Verification items for the finished model (mm, model axes). Coordinates: 2 decimals unless noted, no trailing zeros. Loops run counter-clockwise (first coordinate to the right, second up) from the corner with the lowest first, then second, coordinate; pieces in that order, holes last. Notation, with made-up numbers: (34.25, 61) - (73.25, 61) arc R18 ccw to (73.25, 81) - close; hole circle Ø6 at (61.25, 77). An arc over 180 degrees is marked (long way). One line per item, written item: value. Start each with the question number.
(1) Section check C-C (y = 0). Record the boundary of the cut face in (x, z).
(2) Draft check along X on faces 1 (the face through (-1, -35, 1)), 2 (the face through (-34.136, -1.187, 1.521)), 3 (the face through (-22.387, 18, 2)). Enter one of: +X half, -X half, draft (parallel to the pull), parting line (faces both ways), or undercut.
(3) Thickness scan on probe 1 along X at (y, z) = (-16.5, 0.85); probe 2 along Y at (x, z) = (-37, 1.05); probe 3 along Y at (x, z) = (0, 1.9). Record the ranges inside material, lowest first. Write a range as [from, to].
(4) Section check D-D (x = -32.5). Record the boundary of the cut face in (y, z), plus the area to 3 significant figures.
(5) Section check B-B (x = 13). Record the boundary of the cut face in (y, z), plus the area to 3 significant figures.
(6) Section check A-A (x = 31.5). Record the boundary of the cut face in (y, z).
(7) Gauge pin test, flat ends, axial feed: P1, Ø8, axis at x = -0.5, y = 8.5, coming from the -Z side; P2, Ø3.5, axis at x = -37, y = 0, coming from the +Z side. Record the tip position at first contact, or that the pin passes through.
```python
from build123d import *

# Parameters (mm, degrees)
SKETCH1_W               = 100
SKETCH1_H               = 70
BOSS_EXTRUDE1_DEPTH     = 3
SKETCH2_R               = 3.1
CUT_EXTRUDE1_DEPTH      = 62.10646447
SKETCH3_R               = 1.5
CUT_EXTRUDE2_DEPTH      = 62.10646447
MIRROR2_COPY_1_SKETCH_R = 1.5
MIRROR2_COPY_1_DEPTH    = 62.10646447
CUT_EXTRUDE3_DEPTH      = 62.10646447


with BuildPart() as part:
    # Sketch1 → Boss-Extrude1 (new body)
    with BuildSketch(Plane.XY):
        Rectangle(SKETCH1_W, SKETCH1_H)
    extrude(amount=BOSS_EXTRUDE1_DEPTH)

    # Sketch2 → Cut-Extrude1 (cut, through all)
    with BuildSketch(Plane.XY.offset(3)):
        with Locations((-17, 0)):
            Circle(SKETCH2_R)
        with Locations((-37, 0)):
            Circle(SKETCH2_R)
        with Locations((13, 0)):
            Circle(SKETCH2_R)
    extrude(amount=-CUT_EXTRUDE1_DEPTH, mode=Mode.SUBTRACT)

    # Sketch3 → Cut-Extrude2 (cut, through all)
    with BuildSketch(Plane.XY.offset(3)):
        with Locations((-45.644550594, 30.644550594)):
            Circle(SKETCH3_R)
    cut_extrude2 = extrude(amount=-CUT_EXTRUDE2_DEPTH, mode=Mode.SUBTRACT)

    # Mirror1: Cut-Extrude2 across plane
    add(cut_extrude2.mirror(Plane(origin=(0, 0, 0), x_dir=(0, 0, 1), z_dir=(1, 0, 0))), mode=Mode.SUBTRACT)

    # Mirror2: Cut-Extrude2 across plane
    add(cut_extrude2.mirror(Plane.ZX), mode=Mode.SUBTRACT)

    # Mirror2 copy 1 sketch → Mirror2 copy 1 (cut, through all)
    with BuildSketch(Plane(origin=(0, 0, 3), x_dir=(-1, 0, 0), z_dir=(0, 0, 1))):
        with Locations((-45.644550594, 30.644550594)):
            Circle(MIRROR2_COPY_1_SKETCH_R)
    extrude(amount=-MIRROR2_COPY_1_DEPTH, mode=Mode.SUBTRACT)

    # Sketch4 → Cut-Extrude3 (cut, through all)
    with BuildSketch(Plane.XY.offset(3)):
        with BuildLine():
            Line((7.613447212, 28.5), (-11.613447212, 28.5))
            Line((-11.613447212, 28.5), (-11.613447212, 7.946385912))
            ThreePointArc((-11.613447212, 7.946385912), (-11.211126909, 7.658260137), (-10.824188204, 7.34978562))
            Line((-10.824188204, 7.34978562), (6.824188204, 7.34978562))
            ThreePointArc((6.824188204, 7.34978562), (7.211126909, 7.658260137), (7.613447212, 7.946385912))
            Line((7.613447212, 7.946385912), (7.613447212, 28.5))
        make_face()
        with BuildLine():
            Line((43.5, 7.34978562), (43.5, 22.937352481))
            ThreePointArc((43.5, 22.937352481), (39.987696344, 24.987696344), (37.937352481, 28.5))
            Line((37.937352481, 28.5), (18.386552788, 28.5))
            Line((18.386552788, 28.5), (18.386552788, 7.946385912))
            ThreePointArc((18.386552788, 7.946385912), (18.788873091, 7.658260137), (19.175811796, 7.34978562))
            Line((19.175811796, 7.34978562), (43.5, 7.34978562))
        make_face()
        with BuildLine():
            Line((19.175811796, -7.34978562), (43.5, -7.34978562))
            Line((43.5, -7.34978562), (43.5, -22.937352481))
            ThreePointArc((43.5, -22.937352481), (39.987696344, -24.987696344), (37.937352481, -28.5))
            Line((37.937352481, -28.5), (18.386552788, -28.5))
            Line((18.386552788, -28.5), (18.386552788, -7.946385912))
            ThreePointArc((18.386552788, -7.946385912), (18.788873091, -7.658260137), (19.175811796, -7.34978562))
        make_face()
        with BuildLine():
            Line((-22.386552788, 28.5), (-37.937352481, 28.5))
            ThreePointArc((-37.937352481, 28.5), (-39.987696344, 24.987696344), (-43.5, 22.937352481))
            Line((-43.5, 22.937352481), (-43.5, 7.064700984))
            ThreePointArc((-43.5, 7.064700984), (-37.215853678, 9.597572984), (-30.824188204, 7.34978562))
            Line((-30.824188204, 7.34978562), (-23.175811796, 7.34978562))
            ThreePointArc((-23.175811796, 7.34978562), (-22.788873091, 7.658260137), (-22.386552788, 7.946385912))
            Line((-22.386552788, 7.946385912), (-22.386552788, 28.5))
        make_face()
        with BuildLine():
            Line((-37.937352481, -28.5), (-22.386552788, -28.5))
            Line((-22.386552788, -28.5), (-22.386552788, -7.946385912))
            ThreePointArc((-22.386552788, -7.946385912), (-22.788873091, -7.658260137), (-23.175811796, -7.34978562))
            Line((-23.175811796, -7.34978562), (-30.824188204, -7.34978562))
            ThreePointArc((-30.824188204, -7.34978562), (-37.215853678, -9.597572984), (-43.5, -7.064700984))
            Line((-43.5, -7.064700984), (-43.5, -22.937352481))
            ThreePointArc((-43.5, -22.937352481), (-39.987696344, -24.987696344), (-37.937352481, -28.5))
        make_face()
        with BuildLine():
            Line((-11.613447212, -28.5), (7.613447212, -28.5))
            Line((7.613447212, -28.5), (7.613447212, -7.946385912))
            ThreePointArc((7.613447212, -7.946385912), (7.211126909, -7.658260137), (6.824188204, -7.34978562))
            Line((6.824188204, -7.34978562), (-10.824188204, -7.34978562))
            ThreePointArc((-10.824188204, -7.34978562), (-11.211126909, -7.658260137), (-11.613447212, -7.946385912))
            Line((-11.613447212, -7.946385912), (-11.613447212, -28.5))
        make_face()
    extrude(amount=-CUT_EXTRUDE3_DEPTH, mode=Mode.SUBTRACT)


solid = part.part
```
Responses:
1. outline: (-50, 0) - (-40.1, 0) - (-40.1, 3) - (-50, 3) - close; (-33.9, 0) - (-20.1, 0) - (-20.1, 3) - (-33.9, 3) - close; (-13.9, 0) - (9.9, 0) - (9.9, 3) - (-13.9, 3) - close; (16.1, 0) - (50, 0) - (50, 3) - (16.1, 3) - close
2. face 1: draft
2. face 2: undercut
2. face 3: undercut
3. probe 1: x = [-50, -43.5], [-22.39, -11.61], [7.61, 18.39], [43.5, 50]
3. probe 2: y = [-35, -28.5], [-9.6, -3.1], [3.1, 9.6], [28.5, 35]
3. probe 3: y = [-35, -28.5], [-7.35, 7.35], [28.5, 35]
4. outline: (-35, 0) - (-28.5, 0) - (-28.5, 3) - (-35, 3) - close; (-8.48, 0) - (8.48, 0) - (8.48, 3) - (-8.48, 3) - close; (28.5, 0) - (35, 0) - (35, 3) - (28.5, 3) - close
4. area: 89.9 mm²
5. outline: (-35, 0) - (-3.1, 0) - (-3.1, 3) - (-35, 3) - close; (3.1, 0) - (35, 0) - (35, 3) - (3.1, 3) - close
5. area: 191 mm²
6. outline: (-35, 0) - (-28.5, 0) - (-28.5, 3) - (-35, 3) - close; (-7.35, 0) - (7.35, 0) - (7.35, 3) - (-7.35, 3) - close; (28.5, 0) - (35, 0) - (35, 3) - (28.5, 3) - close
7. P1: stops at z = 0
7. P2: passes through
